Verification items for the finished model (mm, model axes). A direction names the side the tool comes from. Round coordinates to 2 decimals unless told otherwise and drop trailing zeros. Order: outer loops, then holes, each group sorted by start corner. A loop starts at its lowest first (then second) coordinate and runs counter-clockwise, first axis right, second up. Notation, with made-up numbers: (52.25, 56.25) -> (56.25, 56.25) arc R22 ccw to (56.25, 92.25) -> close; hole circle Ø6 at (-24, 67). An arc over 180 degrees is marked (long way). Put each result on its own line as item: value.
from build123d import *

# Parameters (mm, degrees)
F0_W     = 82.1346251114
F0_H     = 41.4849454792
F0_W_2   = 78.0127522687
F0_H_2   = 40.7947400829
F1_DEPTH = 800
F2_W     = 57.8707195818
F2_H     = 25.6879590452
F2_W_2   = 58.3450756967
F2_H_2   = 24.2649074644
F2_W_3   = 48.8580688834
F2_W_4   = 55.0246089697
F2_H_3   = 24.7392579913
F2_W_5   = 47.9093492031
F3_DEPTH = 800


with BuildPart() as f1:
    # F0 (on Front) → F1 (new body)
    with BuildSketch(Plane.XZ):
        Polygon((28.1532571296, 21.6244365409), (-56.7655850202, 21.6244365409), (-56.7655850202, -36.0090098664), (28.1532571296, -36.0090098664), (28.1532571296, 5.4759356128), align=None)
        with Locations((69.2205696853, -15.2665371268)):
            Rectangle(F0_W, F0_H)
        Polygon((110.287882241, 21.6244365409), (110.287882241, 5.4759356128), (110.287882241, -36.0090098664), (180.1719170811, -36.0090098664), (180.1719170811, 4.7857302164), (180.1719170811, 21.6244365409), align=None)
        with Locations((219.1782932154, -15.611639825)):
            Rectangle(F0_W_2, F0_H_2)
        Polygon((258.1846693497, 4.7857302164), (258.1846693497, -36.0090098664), (343.2344149798, -36.0090098664), (343.2344149798, 19.7481851938), (258.1846693497, 19.7481851938), align=None)
    extrude(amount=F1_DEPTH)

    # F2 (on face) → F3 (cut, through all)
    with BuildSketch(Plane.XZ.offset(800)):
        with Locations((-14.3353473395, -12.8439795226)):
            Rectangle(F2_W, F2_H)
        with Locations((71.2848622352, -12.1324537322)):
            Rectangle(F2_W_2, F2_H_2)
        with Locations((146.2321914732, -12.8439795226)):
            Rectangle(F2_W_3, F2_H)
        with Locations((221.4166894555, -12.3696289957)):
            Rectangle(F2_W_4, F2_H_3)
        with Locations((299.9216467142, -12.1324537322)):
            Rectangle(F2_W_5, F2_H_2)
    extrude(amount=-F3_DEPTH, mode=Mode.SUBTRACT)


solid = f1.part
Item 1: Gauge pin test, flat ends, axial feed: pin 1 Ø1.5 at (x, z) = (65.5, 8) entering from -Y; pin 2 Ø4 at (x, y) = (211.5, -412) entering from +Z. Record the tip position at first contact, or that the pin passes through.
Check sheet entries:
pin 1: passes through
pin 2: stops at z = 4.79
Item 2: Release check for a two-part mould opening along X. For faces 1 (the flat face through (140, -800, -26)), 2 (the flat face through (-15, -406, -25.688)), 3 (the flat face through (-56.766, -394, -7)) record: +X half, -X half, draft (parallel to the pull), parting line (faces both ways), or undercut.
Check sheet entries:
face 1: draft
face 2: undercut
face 3: -X half
Item 3: Section check B-B on y = -53.5. State how many separate pieces and enclosed holes the cut face has, then the cut area to 3 significant figures.
Check sheet entries:
separate pieces: 1
enclosed holes: 5
area: 13,600 mm^2
Item 4: Material ranges on L1, parallel to X at y = -49.5, z = 17.5; L2, parallel to X at y = -334, z = -0.5; L3, parallel to X at y = -212, z = -25, recorded low to high. Write a range as [from, to].
Check sheet entries:
L1: x = [-56.77, 28.15], [110.29, 180.17], [258.18, 343.23]
L2: x = [-56.77, -43.27], [14.6, 42.11], [100.46, 121.8], [170.66, 193.9], [248.93, 275.97], [323.88, 343.23]
L3: x = [-56.77, -43.27], [14.6, 121.8], [170.66, 343.23]
Item 5: Tool access check on faces 4 (the flat face through (14.6, -406, -13)), 5 (the flat face through (140, 0, -26)), 6 (the flat face through (69, -394, 5.476)). Record the directions out of +Z, -Z, +X, -X, +Y, -Y that give a thin tool (end or side, any length) a straight path to the whole face; none if there is none.
Check sheet entries:
face 4: +Y, -Y
face 5: +Z, -Z, +X, -X, +Y
face 6: +Z, +Y, -Y
Item 6: Section check A-A on x = 313.5. Record the boundary of the cut face in (y, z).
Check sheet entries:
outline: (-800, -36.01) -> (0, -36.01) -> (0, -24.26) -> (-800, -24.26) -> close; (-800, 0) -> (0, 0) -> (0, 19.75) -> (-800, 19.75) -> close
Item 7: Section check C-C on x = -24. Record the boundary of the cut face in (y, z).
Check sheet entries:
outline: (-800, -36.01) -> (0, -36.01) -> (0, -25.69) -> (-800, -25.69) -> close; (-800, 0) -> (0, 0) -> (0, 21.62) -> (-800, 21.62) -> close
